```python
from build123d import *

# Parameters (mm, degrees)
ESQUISSE1_R                  = 9
BOSS_EXTRU_1_DEPTH           = 4
BOSS_EXTRU_2_DEPTH           = 5
ENL_V_MAT_EXTRU_1_DEPTH      = 4
ENL_V_MAT_EXTRU_2_DEPTH      = 3
ENL_V_MAT_EXTRU_2_DEPTH_BACK = 12
ESQUISSE4_R                  = 1.6
BOSS_EXTRU_3_DEPTH           = 3
BOSS_EXTRU_3_DEPTH_BACK      = 8
ESQUISSE5_W                  = 12
ESQUISSE5_H                  = 2.3
ENL_V_MAT_EXTRU_3_DEPTH      = 11
ESQUISSE7_R                  = 1.6
ENL_V_MAT_EXTRU_4_DEPTH      = 11


with BuildPart() as part:
    # Esquisse1 → Boss.-Extru.1 (new body)
    with BuildSketch(Plane(origin=(0, 0, 0), x_dir=(1, 0, 0), z_dir=(0, 1, 0))):
        with Locations(Location((0, 0, 0), (0, 0, 270))):
            Circle(ESQUISSE1_R)
    extrude(amount=BOSS_EXTRU_1_DEPTH)

    # Esquisse2 → Boss.-Extru.2 (add)
    with BuildSketch(Plane(origin=(0, 4, 0), x_dir=(1, 0, 0), z_dir=(0, 1, 0))):
        with BuildLine():
            Line((0, 2.85), (28, 2.85))
            Line((28, 2.85), (40, 2.85))
            Line((40, 2.85), (41.582547561, 1.321751585))
            Line((41.582547561, 1.321751585), (41.582547561, -6.678248415))
            Line((41.582547561, -6.678248415), (29.582547561, -6.678248415))
            Line((29.582547561, -6.678248415), (29.582547561, -4.378248415))
            Line((29.582547561, -4.378248415), (28, -2.85))
            Line((28, -2.85), (0, -2.85))
            add(Edge.make_bspline(
                [(0, 2.85), (-1.583763235, 2.944784931), (-4.146375178, 0.014422281), (-1.543874763, -2.966253476), (0, -2.85)],
                knots=[0, 0, 0, 0, 0.500311959, 1, 1, 1, 1], degree=3))
        make_face()
    extrude(amount=BOSS_EXTRU_2_DEPTH)

    # Esquisse3 → Enlèv. mat.-Extru.1 (cut)
    with BuildSketch(Plane.XZ):
        Polygon((0.351449311, 8.993135348), (0.513444021, 7.221842901), (1.577304258, 7.034102859), (2.276601179, 8.707300791), (1.416805586, 9.582955874), align=None)
        Polygon((3.344118704, 6.386185235), (4.452643151, 7.821378969), (3.848780595, 8.889728302), (2.667068669, 8.595739917), (2.365099324, 6.84287548), align=None)
        Polygon((4.883036987, 5.30305964), (6.325244851, 6.402443094), (6.018467567, 7.590680437), (4.800931705, 7.612559016), (4.055577016, 5.997577404), align=None)
        Polygon((6.089184369, 3.858539294), (7.766791567, 4.547191304), (7.77800592, 5.774340245), (6.607619179, 6.110594798), (5.469673837, 4.743554339), align=None)
        Polygon((6.880363898, 2.151065872), (8.679044273, 2.382055941), (9.007486024, 3.564488307), (7.964008326, 4.192203643), (6.511021425, 3.166265885), align=None)
        Polygon((7.202657999, 0.297000866), (8.999834455, 0.054587401), (9.62312084, 1.111722382), (8.777663467, 1.988120738), (7.108653663, 1.373201643), align=None)
        Polygon((7.034102859, -1.577304258), (8.707300791, -2.276601179), (9.582955874, -1.416805586), (8.993135348, -0.351449311), (7.221842901, -0.513444021), align=None)
        Polygon((6.386185235, -3.344118704), (7.821378969, -4.452643151), (8.889728302, -3.848780595), (8.595739917, -2.667068669), (6.84287548, -2.365099324), align=None)
        Polygon((5.30305964, -4.883036987), (6.402443094, -6.325244851), (7.590680437, -6.018467567), (7.612559016, -4.800931705), (5.997577404, -4.055577016), align=None)
        Polygon((3.858539294, -6.089184369), (4.547191304, -7.766791567), (5.774340245, -7.77800592), (6.110594798, -6.607619179), (4.743554339, -5.469673837), align=None)
        Polygon((2.151065872, -6.880363898), (2.382055941, -8.679044273), (3.564488307, -9.007486024), (4.192203643, -7.964008326), (3.166265885, -6.511021425), align=None)
        Polygon((0.297000866, -7.202657999), (0.054587401, -8.999834455), (1.111722382, -9.62312084), (1.988120738, -8.777663467), (1.373201643, -7.108653663), align=None)
        Polygon((-1.577304258, -7.034102859), (-2.276601179, -8.707300791), (-1.416805586, -9.582955874), (-0.351449311, -8.993135348), (-0.513444021, -7.221842901), align=None)
        Polygon((-3.344118704, -6.386185235), (-4.452643151, -7.821378969), (-3.848780595, -8.889728302), (-2.667068669, -8.595739917), (-2.365099324, -6.84287548), align=None)
        Polygon((-4.883036987, -5.30305964), (-6.325244851, -6.402443094), (-6.018467567, -7.590680437), (-4.800931705, -7.612559016), (-4.055577016, -5.997577404), align=None)
        Polygon((-6.089184369, -3.858539294), (-7.766791567, -4.547191304), (-7.77800592, -5.774340245), (-6.607619179, -6.110594798), (-5.469673837, -4.743554339), align=None)
        Polygon((-6.880363898, -2.151065872), (-8.679044273, -2.382055941), (-9.007486024, -3.564488307), (-7.964008326, -4.192203643), (-6.511021425, -3.166265885), align=None)
        Polygon((-7.202657999, -0.297000866), (-8.999834455, -0.054587401), (-9.62312084, -1.111722382), (-8.777663467, -1.988120738), (-7.108653663, -1.373201643), align=None)
        Polygon((-7.034102859, 1.577304258), (-8.707300791, 2.276601179), (-9.582955874, 1.416805586), (-8.993135348, 0.351449311), (-7.221842901, 0.513444021), align=None)
        Polygon((-6.386185235, 3.344118704), (-7.821378969, 4.452643151), (-8.889728302, 3.848780595), (-8.595739917, 2.667068669), (-6.84287548, 2.365099324), align=None)
        Polygon((-5.30305964, 4.883036987), (-6.402443094, 6.325244851), (-7.590680437, 6.018467567), (-7.612559016, 4.800931705), (-5.997577404, 4.055577016), align=None)
        Polygon((-3.858539294, 6.089184369), (-4.547191304, 7.766791567), (-5.774340245, 7.77800592), (-6.110594798, 6.607619179), (-4.743554339, 5.469673837), align=None)
        Polygon((-2.151065872, 6.880363898), (-2.382055941, 8.679044273), (-3.564488307, 9.007486024), (-4.192203643, 7.964008326), (-3.166265885, 6.511021425), align=None)
        Polygon((-0.297000866, 7.202657999), (-0.054587401, 8.999834455), (-1.111722382, 9.62312084), (-1.988120738, 8.777663467), (-1.373201643, 7.108653663), align=None)
    extrude(amount=-ENL_V_MAT_EXTRU_1_DEPTH, mode=Mode.SUBTRACT)

    # Esquisse4 → Enlèv. mat.-Extru.2 (cut, two sides: drawn at the far end of the back side and taken through both)
    with BuildSketch(Plane(origin=(0, 9, 0), x_dir=(1, 0, 0), z_dir=(0, 1, 0)).offset(-ENL_V_MAT_EXTRU_2_DEPTH_BACK)):
        with Locations(Location((0, 0, 0), (0, 0, 90))):
            Circle(ESQUISSE4_R)
    extrude(amount=ENL_V_MAT_EXTRU_2_DEPTH + ENL_V_MAT_EXTRU_2_DEPTH_BACK, mode=Mode.SUBTRACT)

    # Esquisse5 → Boss.-Extru.3 (add, two sides: drawn at the far end of the back side and taken through both)
    with BuildSketch(Plane(origin=(0, 9, 0), x_dir=(1, 0, 0), z_dir=(0, 1, 0)).offset(-BOSS_EXTRU_3_DEPTH_BACK)):
        with Locations((35.582547561, -5.528248415)):
            Rectangle(ESQUISSE5_W, ESQUISSE5_H)
    extrude(amount=BOSS_EXTRU_3_DEPTH + BOSS_EXTRU_3_DEPTH_BACK)

    # Esquisse6 → Enlèv. mat.-Extru.3 (cut)
    with BuildSketch(Plane(origin=(0, 12, 0), x_dir=(1, 0, 0), z_dir=(0, 1, 0))):
        Polygon((41.30726734, -6.678248415), (41.004659891, -6.028248415), (40.65726734, -6.678248415), (41.004659891, -7.030774788), align=None)
        Polygon((40.32726734, -6.678248415), (40.024659891, -6.028248415), (39.67726734, -6.678248415), (40.024659891, -7.030774788), align=None)
        Polygon((39.34726734, -6.678248415), (39.044659891, -6.028248415), (38.69726734, -6.678248415), (39.044659891, -7.030774788), align=None)
        Polygon((38.36726734, -6.678248415), (38.064659891, -6.028248415), (37.71726734, -6.678248415), (38.064659891, -7.030774788), align=None)
        Polygon((37.38726734, -6.678248415), (37.084659891, -6.028248415), (36.73726734, -6.678248415), (37.084659891, -7.030774788), align=None)
        Polygon((36.40726734, -6.678248415), (36.104659891, -6.028248415), (35.75726734, -6.678248415), (36.104659891, -7.030774788), align=None)
        Polygon((35.42726734, -6.678248415), (35.124659891, -6.028248415), (34.77726734, -6.678248415), (35.124659891, -7.030774788), align=None)
        Polygon((34.44726734, -6.678248415), (34.144659891, -6.028248415), (33.79726734, -6.678248415), (34.144659891, -7.030774788), align=None)
        Polygon((33.46726734, -6.678248415), (33.164659891, -6.028248415), (32.81726734, -6.678248415), (33.164659891, -7.030774788), align=None)
        Polygon((32.48726734, -6.678248415), (32.184659891, -6.028248415), (31.83726734, -6.678248415), (32.184659891, -7.030774788), align=None)
        Polygon((31.50726734, -6.678248415), (31.204659891, -6.028248415), (30.85726734, -6.678248415), (31.204659891, -7.030774788), align=None)
        Polygon((30.52726734, -6.678248415), (30.224659891, -6.028248415), (29.87726734, -6.678248415), (30.224659891, -7.030774788), align=None)
    extrude(amount=-ENL_V_MAT_EXTRU_3_DEPTH, mode=Mode.SUBTRACT)

    # Esquisse7 → Enlèv. mat.-Extru.4 (cut)
    with BuildSketch(Plane(origin=(0, 9, 0), x_dir=(1, 0, 0), z_dir=(0, 1, 0))):
        with Locations(Location((38, 0, 0), (0, 0, 270))):
            Circle(ESQUISSE7_R)
    extrude(amount=-ENL_V_MAT_EXTRU_4_DEPTH, mode=Mode.SUBTRACT)


solid = part.part
```
Geometry: final body of the model. Coordinates: model frame, mm. A direction names the side the tool comes from. Give positions to 0.01 mm unless a question says otherwise; leave off trailing zeros. Loops run counter-clockwise (first coordinate to the right, second up) from the corner with the lowest first, then second, coordinate; pieces in that order, holes last. Notation, with made-up numbers: (-3, -22) -> (44, -22) arc R18 ccw to (44, 7) -> close; hole circle Ø2 at (3.25, 21). An arc over 180 degrees is marked (long way). Return JSON: item names as keys, results as strings.
Item 1: Access query for faces 5 (the flat face through (5.775, 1.972, 4.307)), 6 (the flat face through (-5.845, 1.972, 5.594)), 7 (the flat face through (7.859, 1.972, -1.922)), 8 (the flat face through (-1.7, 2, 8)). Directions: +Z, -Z, +X, -X, +Y, -Y. A direction counts if a zero-diameter tool reaches every point of the face in a straight line with its end or side. Return the directions, or none.
Filled in:
{"face 5": "+Y, -Y", "face 6": "-X, +Y, -Y", "face 7": "+X, -Y", "face 8": "+Z, +Y, -Y"}
Item 2: Pin query (flat end, axial travel): P1, Ø5, axis at x = -4, z = -2, coming from the +Y side; P2, Ø3, axis at x = 0, z = 0, coming from the -Y side; P3, Ø6, axis at x = 36.5, z = -1, coming from the -Y side; P4, Ø4, axis at x = 16.5, y = 6, coming from the +Z side. Return the tip coordinate at first contact, or that it passes through.
Filled in:
{"P1": "y = 9", "P2": "through", "P3": "y = 4", "P4": "z = 2.85"}
Item 3: Section A-A, the plane y = 6.75. Count the separate pieces of the cut face and the enclosed holes in it, plus the area to 3 significant figures.
Filled in:
{"separate pieces": "1", "enclosed holes": "2", "area": "277 mm^2"}
Item 4: Mould query, pull axis X, two halves, no side actions, for faces 1 (the flat face through (35.5, 12, 5.5)), 2 (the flat face through (6.92, 1.97, 4.2)), 3 (the flat face through (7.25, 1.97, 3.69)), 4 (the flat face through (-6.05, 1.97, -5.44)). Classes: released by +X, released by -X, zero draft, split by the parting line, or undercut.
Filled in:
{"face 1": "zero draft", "face 2": "undercut", "face 3": "released by +X", "face 4": "released by -X"}
Item 5: Section B-B, the plane x = 17. Output: boundary loops of the cut face in (y, z), plus the area to 3 significant figures.
Filled in:
{"outline": "(4, -2.85) -> (9, -2.85) -> (9, 2.85) -> (4, 2.85) -> close", "area": "28.5 mm^2"}
Item 6: Line query: line 1 (X direction, y = 6.6, z = 0); line 2 (X direction, y = 8, z = -1.25); line 3 (Y direction, x = -2.5, z = -4.5). Output: solid intervals per line, ascending.
Filled in:
{"line 1": "-2.86 to -1.6, 1.6 to 36.4, 39.6 to 41.58", "line 2": "-2.56 to -1, 1 to 37, 39 to 41.58", "line 3": "0 to 4"}
